CAD build for the part. Positions are in the model's coordinates, mm. A direction names the side the tool comes from. Give positions to 0.01 mm unless a question says otherwise; leave off trailing zeros. Order: outer loops, then holes, each group sorted by start corner. A loop starts at its lowest first (then second) coordinate and runs counter-clockwise, first axis right, second up. Notation, with made-up numbers: M 75,60.5 L 93,60.5 A10 cw 93,77.5 Z; hole C 55,26.25 d10. An arc over 180 degrees is marked long. Put each result on its own line as item: value. Start each with the question number.
1) Tool access for faces 1 (the face through (-327, 70, 3)), 2 (the face through (-285, 174, 3)), 3 (the face through (-232, 3, 3)), 4 (the face through (-3, 130, 3)), 5 (the face through (-270, 3, 3)): list every direction of +Z, -Z, +X, -X, +Y, -Y with a clear straight run to the whole face (end or side of a thin tool).
2) Cut at A-A (x = -108.5). Write the cut outline in (y, z), and give its area (3 significant figures).
3) Cut at B-B (y = 101.5). Write the cut outline in (x, z).
4) Pin check, flat tips, straight feed: pin 1 (1.8 mm diameter, centred on x = -153, z = 3.5, fed in from -Y); pin 2 (1.8 mm diameter, centred on x = -151.5, z = 2, fed in from +Y); pin 3 (1.8 mm diameter, centred on y = 80.5, z = 2, fed in from +X). Stop position of each tip, or through.
5) Two-plate mould, pull along Y, no slides. Class faces 6 (the face through (-166, 6, 3)), 7 (the face through (-327, 110, 3)), 8 (the face through (-3, 70, 3)), 9 (the face through (-330, 120, 3)): released by +Y, released by -Y, zero draft, split by the parting line, or undercut.
6) Drill centre lines: line 1 (X direction, y = 169, z = 4.85); line 2 (Y direction, x = -311.5, z = 4.2); line 3 (Y direction, x = -106, z = 2.05). Where is each one in solid material? Low to high. Write a range as [from, to].
```python
from build123d import *

# Parameters (mm, degrees)
ESQUISSE1_W             = 330
ESQUISSE1_H             = 180
BOSS_EXTRU_1_DEPTH      = 6
ESQUISSE2_W             = 6
ESQUISSE2_H             = 40
ESQUISSE2_W_2           = 80
ESQUISSE2_H_2           = 6
ESQUISSE2_W_3           = 134
ENL_V_MAT_EXTRU_1_DEPTH = 376.946804748


with BuildPart() as part:
    # Esquisse1 → Boss.-Extru.1 (new body)
    with BuildSketch(Plane.XY):
        with Locations((-165, 90)):
            Rectangle(ESQUISSE1_W, ESQUISSE1_H)
    extrude(amount=BOSS_EXTRU_1_DEPTH)

    # Esquisse2 → Enlèv. mat.-Extru.1 (cut, through all)
    with BuildSketch(Plane.XY.offset(6)):
        Polygon((-330, 180), (-330, 130), (-324, 130), (-324, 174), (-244, 174), (-244, 180), align=None)
        Polygon((-330, 0), (-330, 50), (-324, 50), (-324, 6), (-270, 6), (-270, 0), align=None)
        with Locations((-327, 90)):
            Rectangle(ESQUISSE2_W, ESQUISSE2_H)
        Polygon((0, 180), (0, 130), (-6, 130), (-6, 174), (-86, 174), (-86, 180), align=None)
        Polygon((0, 0), (0, 50), (-6, 50), (-6, 6), (-60, 6), (-60, 0), align=None)
        with Locations((-3, 90)):
            Rectangle(ESQUISSE2_W, ESQUISSE2_H)
        with Locations((-165, 177)):
            Rectangle(ESQUISSE2_W_2, ESQUISSE2_H_2)
        with Locations((-165, 3)):
            Rectangle(ESQUISSE2_W_3, ESQUISSE2_H_2)
    extrude(amount=-ENL_V_MAT_EXTRU_1_DEPTH, mode=Mode.SUBTRACT)


solid = part.part
```
Solution:
1. face 1: +Z, -Z, -X
1. face 2: +Z, -Z, -X, +Y
1. face 3: +Z, -Z, -Y
1. face 4: +Z, -Z, +X, +Y
1. face 5: +Z, -Z, -X, -Y
2. outline: M 6,0 L 180,0 L 180,6 L 6,6 Z
2. area: 1,040 mm²
3. outline: M -324,0 L -6,0 L -6,6 L -324,6 Z
4. pin 1: y = 6
4. pin 2: y = 174
4. pin 3: x = -6
5. face 6: released by -Y
5. face 7: undercut
5. face 8: undercut
5. face 9: zero draft
6. line 1: [-324, -6]
6. line 2: [6, 174]
6. line 3: [6, 180]
